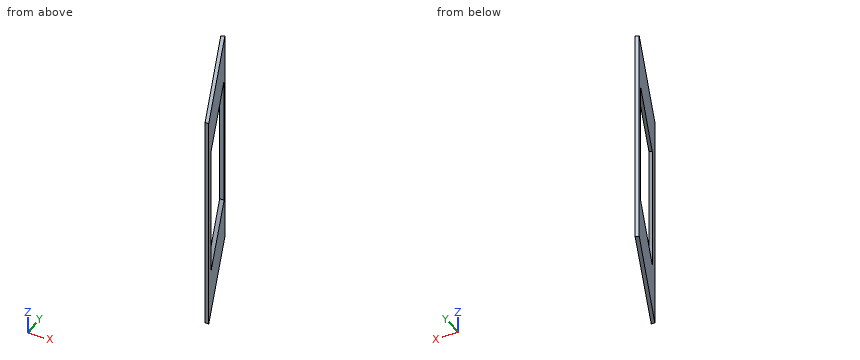
```python
from build123d import *

# Parameters (mm, degrees)
BOSS_EXTRU_1_DEPTH      = 600
ESQUISSE2_W             = 338.746
ESQUISSE2_H             = 271
ENL_V_MAT_EXTRU_1_DEPTH = 10
ENL_V_MAT_EXTRU_1_TAPER = -45


with BuildPart() as part:
    # Esquisse1 → Boss.-Extru.1 (new body)
    with BuildSketch(Plane.XY):
        Polygon((235.606802378, 81.334991463), (103.65574387, 410.044643603), (112.874448857, 413.919624682), (245.500189591, 81.334991463), align=None)
    extrude(amount=BOSS_EXTRU_1_DEPTH)

    # Esquisse2 → Enlèv. mat.-Extru.1 (cut)
    with BuildSketch(Plane(origin=(231.028658646, 92.739826335, 0), x_dir=(0, 0, 1), z_dir=(-0.928021166, -0.37252747, 0))):
        with Locations((300.232670333, 181.16149611)):
            Rectangle(ESQUISSE2_W, ESQUISSE2_H)
    extrude(amount=-ENL_V_MAT_EXTRU_1_DEPTH, taper=ENL_V_MAT_EXTRU_1_TAPER, mode=Mode.SUBTRACT)


solid = part.part
```
Geometry check sheet. Reference: the model listing, model coordinates, mm. Give positions to 0.01 mm unless a question says otherwise; leave off trailing zeros. Order: outer loops, then holes, each group sorted by start corner. A loop starts at its lowest first (then second) coordinate and runs counter-clockwise, first axis right, second up.
1. Section check A-A, the plane z = 547. Enter the section's corners in (x, y) (3 decimals), and give its area (3 significant figures).
2. Thickness scan on L1, parallel to Z at x = 159, y = 283.5; L2, parallel to X at y = 323.5, z = 59; L3, parallel to X at y = 292, z = 125.5. Record the ranges inside material, lowest first.
3. Section check B-B, the plane y = 123. Enter the section's corners in (x, z), and give its area (3 significant figures).
Values follow:
1. outline: (103.656, 410.045) - (235.607, 81.335) - (245.5, 81.335) - (112.874, 413.92) - close
1. area: 3,420 mm2
2. L1: z = 0 to 126.64, 473.82 to 600
2. L2: x = 138.4 to 148.93
2. L3: x = 151.04 to 156.82
3. outline: (218.88, 0) - (228.89, 0) - (228.89, 600) - (218.88, 600) - close
3. area: 6,000 mm2
